```python
from build123d import *

# Parameters (mm, degrees)
SKETCH_1_W              = 10
SKETCH_1_H              = 20
EXTRUDE_1_DEPTH         = 3
HOLE_WIZARD_2_2_2_2_1_D = 2.2
SKETCH_5_W              = 20
SKETCH_5_H              = 40
EXTRUDE_2_DEPTH         = 80
CUT_EXTRUDE_1_REACH     = 107
SKETCH_6_W              = 74
SKETCH_6_H              = 37
HOLE_WIZARD_2_2_2_2_2_D = 2.2
FILLET_1_R              = 0.7


with BuildPart() as part:
    # 草图1 → 凸台-拉伸1 (new body)
    with BuildSketch(Plane(origin=(0, 0, 0), x_dir=(1, 0, 0), z_dir=(0, 1, 0))):
        Rectangle(SKETCH_1_W, SKETCH_1_H)
    extrude_1 = extrude(amount=EXTRUDE_1_DEPTH)

    # Ø2.2 (2.2) 直径孔1 (through all)
    with Locations(Plane(origin=(0, 3, 0), x_dir=(1, 0, 0), z_dir=(0, 1, 0))):
        with Locations((0, 5), (0, -5)):
            hole_wizard_2_2_2_2_1 = Hole(HOLE_WIZARD_2_2_2_2_1_D / 2)

    # 草图5 → 凸台-拉伸2 (add)
    with BuildSketch(Plane(origin=(5, 0, 0), x_dir=(0, 0, -1), z_dir=(1, 0, 0))):
        with Locations((0, 20)):
            Rectangle(SKETCH_5_W, SKETCH_5_H)
    extrude(amount=EXTRUDE_2_DEPTH)

    # 镜向1: 凸台-拉伸1, Ø2.2 (2.2) 直径孔1 across plane
    add(extrude_1.mirror(Plane.ZY.offset(-45)))
    add(hole_wizard_2_2_2_2_1.mirror(Plane.ZY.offset(-45)), mode=Mode.SUBTRACT)

    # 草图6 → 切除-拉伸1 (cut, up to next)
    with BuildSketch(Plane.XY.offset(10), mode=Mode.PRIVATE) as cut_extrude_1_sk1:
        with Locations((45, 18.5)):
            Rectangle(SKETCH_6_W, SKETCH_6_H)
    cut_extrude_1_tool1 = extrude(cut_extrude_1_sk1.sketch, amount=-CUT_EXTRUDE_1_REACH, mode=Mode.PRIVATE) & part.part
    add(cut_extrude_1_tool1.solids().sort_by_distance((45, 18.5, 10))[0], mode=Mode.SUBTRACT)

    # Ø2.2 (2.2) 直径孔2 (through all)
    with Locations(Plane(origin=(0, 40, 0), x_dir=(1, 0, 0), z_dir=(0, 1, 0))):
        with Locations((20.5, 0), (69.5, 0)):
            Hole(HOLE_WIZARD_2_2_2_2_2_D / 2)

    # 圆角1
    fillet_1_edges = [part.edges().sort_by_distance(p)[0] for p in [
        (5, 3, 0),
        (0, 3, -10),
        (5, 21.5, 10),
        (45, 40, 10),
        (5, 21.5, -10),
        (5, 40, 0),
        (45, 40, -10),
        (85, 21.5, 10),
        (85, 40, 0),
        (85, 21.5, -10),
        (95, 3, 0),
        (90, 3, -10),
        (85, 3, 0),
        (90, 3, 10),
        (-5, 3, 0),
        (88.5, 0, -10),
        (1.5, 0, 10),
        (1.5, 0, -10),
        (88.5, 0, 10),
        (8, 0, 0),
        (8, 37, 0),
        (82, 37, 0),
        (82, 0, 0),
        (8, 18.5, 10),
        (82, 18.5, 10),
        (45, 37, 10),
        (8, 18.5, -10),
        (45, 37, -10),
        (82, 18.5, -10),
        (0, 3, 10),
    ]]
    fillet(fillet_1_edges, radius=FILLET_1_R)


solid = part.part
```
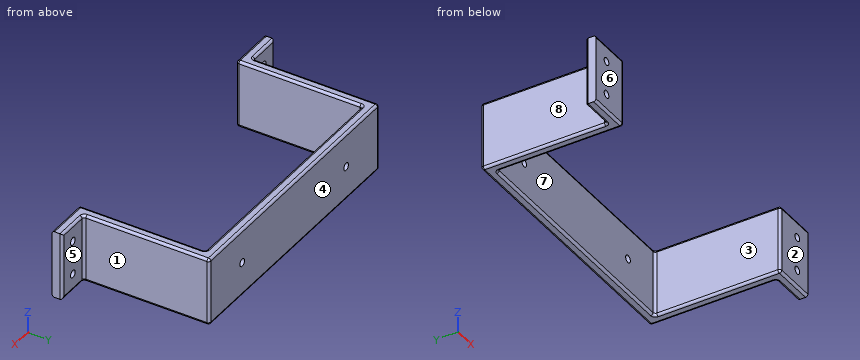
Source: CAD feature listing. Evaluate the final solid. Frame: model axes, mm. Face numbers are marked on the shaded views. A direction names the side the tool comes from. Round coordinates to 2 decimals unless told otherwise and drop trailing zeros. Loops run counter-clockwise (first coordinate to the right, second up) from the corner with the lowest first, then second, coordinate; pieces in that order, holes last. Notation, with made-up numbers: M -31,34 L 22,34 A29 ccw 22,65 Z; hole C -10.5,13.25 d3. An arc over 180 degrees is marked long. Use a Markdown table: item, result. Add a question column.
1. Section query D-D on x = 0. Return the cut outline in (y, z).
2. Line query: line 1 (Z direction, x = 0, y = 1.8); line 2 (X direction, y = 20.5, z = -0.25); line 3 (Z direction, x = 20.5, y = 39.05). Output: solid intervals per line, ascending.
3. Mould query, pull axis X, two halves, no side actions, for the marked faces 1, 2 and 3. Classes: pulls with the +X half, pulls with the -X half, needs draft (parallel to the pull), parting line crosses it, or undercut.
4. Section query B-B on z = -5. Give the number of separate pieces and of enclosed holes in the cut face, then the cut area to 3 significant figures.
5. Section query C-C on x = 20.5. Return the cut outline in (y, z).
6. Reachability of the marked faces 4, 5, 6, 7 and 8 from +Z, -Z, +X, -X, +Y, -Y: full face, straight path, thin tool, end or side. Return the list, or none.
7. Section query A-A on y = 34.5. Return the cut outline in (x, z).
8. Contact query for flat-ended pins moving along their axis: P1, Ø5.5, axis at y = 20, z = 0.5, coming from the +X side; P2, Ø1.3, axis at x = 20.5, z = 0, coming from the +Y side; P3, Ø5.5, axis at y = 27, z = -1, coming from the -X side; P4, Ø3, axis at x = 69.5, z = 0, coming from the -Y side. Output: stop coordinate, or through.
Reported:
| question | item | result |
|---|---|---|
| 1 | outline | M 0,-9.3 A0.7 ccw 0.7,-10 L 2.3,-10 A0.7 ccw 3,-9.3 L 3,-6.1 L 0,-6.1 Z; M 0,-3.9 L 3,-3.9 L 3,3.9 L 0,3.9 Z; M 0,6.1 L 3,6.1 L 3,9.3 A0.7 ccw 2.3,10 L 0.7,10 A0.7 ccw 0,9.3 Z |
| 2 | line 1 | z = -10 to -6.1, -3.9 to 3.9, 6.1 to 10 |
| 2 | line 2 | x = 5 to 8, 82 to 85 |
| 2 | line 3 | z = -10 to -1.1, 1.1 to 10 |
| 3 | face 1 | pulls with the +X half |
| 3 | face 2 | needs draft |
| 3 | face 3 | undercut |
| 4 | separate pieces | 3 |
| 4 | enclosed holes | 0 |
| 4 | area | 509 mm² |
| 5 | outline | M 37,-9.3 A0.7 ccw 37.7,-10 L 39.3,-10 A0.7 ccw 40,-9.3 L 40,-1.1 L 37,-1.1 Z; M 37,1.1 L 40,1.1 L 40,9.3 A0.7 ccw 39.3,10 L 37.7,10 A0.7 ccw 37,9.3 Z |
| 6 | face 4 | +Z, -Z, +X, -X, +Y |
| 6 | face 5 | +Z, -Z, +X, +Y |
| 6 | face 6 | +Z, -Z, +X, -X, -Y |
| 6 | face 7 | +Z, -Z, -Y |
| 6 | face 8 | +Z, -Z, -X, +Y |
| 7 | outline | M 5,-9.3 A0.7 ccw 5.7,-10 L 7.3,-10 A0.7 ccw 8,-9.3 L 8,9.3 A0.7 ccw 7.3,10 L 5.7,10 A0.7 ccw 5,9.3 Z; M 82,-9.3 A0.7 ccw 82.7,-10 L 84.3,-10 A0.7 ccw 85,-9.3 L 85,9.3 A0.7 ccw 84.3,10 L 82.7,10 A0.7 ccw 82,9.3 Z |
| 8 | P1 | stops at x = 85 |
| 8 | P2 | passes through |
| 8 | P3 | stops at x = 5 |
| 8 | P4 | stops at y = 37 |
